Work out the finished part from the listing and answer in its coordinate system (mm). A direction names the side the tool comes from. Round coordinates to 2 decimals unless told otherwise and drop trailing zeros. Loops run counter-clockwise (first coordinate to the right, second up) from the corner with the lowest first, then second, coordinate; pieces in that order, holes last. Notation, with made-up numbers: (-12, 66.5) -> (32, 66.5) arc R24 cw to (32, 89.5) -> close; hole circle Ø1 at (74, -16). An arc over 180 degrees is marked (long way). Write item = value, one per line. Start each with the question number.
```python
from build123d import *

# Parameters (mm, degrees)
BOSS_EXTRU_1_DEPTH      = 7.5
ENL_V_MAT_EXTRU_1_DEPTH = 2
ESQUISSE5_R             = 3.25
ENL_V_MAT_EXTRU_2_DEPTH = 144.052645944
ESQUISSE7_R             = 6.5
ENL_V_MAT_EXTRU_3_DEPTH = 144.143492733


with BuildPart() as part:
    # Esquisse2 → Boss.-Extru.1 (new body)
    with BuildSketch(Plane(origin=(0, 0, 0), x_dir=(1, 0, 0), z_dir=(0, 1, 0))):
        with BuildLine():
            Line((79.497474683, -37.071067812), (42.426406871, 0))
            Line((42.426406871, 0), (79.497474683, 37.071067812))
            ThreePointArc((79.497474683, 37.071067812), (79.497474683, 79.497474683), (37.071067812, 79.497474683))
            Line((37.071067812, 79.497474683), (0, 42.426406871))
            Line((0, 42.426406871), (-37.071067812, 79.497474683))
            ThreePointArc((-37.071067812, 79.497474683), (-79.497474683, 79.497474683), (-79.497474683, 37.071067812))
            Line((-79.497474683, 37.071067812), (-42.426406871, 0))
            Line((-42.426406871, 0), (-79.497474683, -37.071067812))
            ThreePointArc((-79.497474683, -37.071067812), (-79.497474683, -79.497474683), (-37.071067812, -79.497474683))
            Line((-37.071067812, -79.497474683), (-30, -72.426406871))
            Line((-30, -72.426406871), (-30, -82.426406871))
            ThreePointArc((-30, -82.426406871), (0, -112.426406871), (30, -82.426406871))
            Line((30, -82.426406871), (30, -72.426406871))
            Line((30, -72.426406871), (37.071067812, -79.497474683))
            ThreePointArc((37.071067812, -79.497474683), (79.497474683, -79.497474683), (79.497474683, -37.071067812))
        make_face()
    extrude(amount=BOSS_EXTRU_1_DEPTH)

    # Esquisse4 → Enlèv. mat.-Extru.1 (cut)
    with BuildSketch(Plane(origin=(0, 0, 0), x_dir=(-1, 0, 0), z_dir=(0, -1, 0))):
        with BuildLine():
            Line((-33.535533906, -33.535533906), (-18.245921943, -18.245921943))
            Line((-18.245921943, -18.245921943), (-28.852523661, -7.639320225))
            Line((-28.852523661, -7.639320225), (-46.53019319, -25.316989755))
            ThreePointArc((-46.53019319, -25.316989755), (-39.575984314, -28.703872332), (-33.535533906, -33.535533906))
        make_face()
        with BuildLine():
            Line((-7.639320225, -28.852523661), (-18.245921943, -18.245921943))
            Line((-18.245921943, -18.245921943), (-33.535533906, -33.535533906))
            ThreePointArc((-33.535533906, -33.535533906), (-28.703872332, -39.575984314), (-25.316989755, -46.53019319))
            Line((-25.316989755, -46.53019319), (-7.639320225, -28.852523661))
        make_face()
        with BuildLine():
            ThreePointArc((-46.53019319, 25.316989755), (-33.535533906, 33.535533906), (-25.316989755, 46.53019319))
            Line((-25.316989755, 46.53019319), (-7.639320225, 28.852523661))
            Line((-7.639320225, 28.852523661), (-28.852523661, 7.639320225))
            Line((-28.852523661, 7.639320225), (-46.53019319, 25.316989755))
        make_face()
        with BuildLine():
            ThreePointArc((25.316989755, 46.53019319), (33.535533906, 33.535533906), (46.53019319, 25.316989755))
            Line((46.53019319, 25.316989755), (28.852523661, 7.639320225))
            Line((28.852523661, 7.639320225), (7.639320225, 28.852523661))
            Line((7.639320225, 28.852523661), (25.316989755, 46.53019319))
        make_face()
        with BuildLine():
            ThreePointArc((46.53019319, -25.316989755), (33.535533906, -33.535533906), (25.316989755, -46.53019319))
            Line((25.316989755, -46.53019319), (7.639320225, -28.852523661))
            Line((7.639320225, -28.852523661), (28.852523661, -7.639320225))
            Line((28.852523661, -7.639320225), (46.53019319, -25.316989755))
        make_face()
    extrude(amount=-ENL_V_MAT_EXTRU_1_DEPTH, mode=Mode.SUBTRACT)

    # Esquisse5 → Enlèv. mat.-Extru.2 (cut, through all)
    with BuildSketch(Plane(origin=(0, 2, 0), x_dir=(-1, 0, 0), z_dir=(0, -1, 0))):
        with Locations(Location((-25.316989755, -25.316989755, 0), (0, 0, 90))):
            Circle(ESQUISSE5_R)
        with Locations(Location((-25.316989755, 25.316989755, 0), (0, 0, 90))):
            Circle(ESQUISSE5_R)
        with Locations(Location((25.316989755, 25.316989755, 0), (0, 0, 90))):
            Circle(ESQUISSE5_R)
        with Locations(Location((25.316989755, -25.316989755, 0), (0, 0, 90))):
            Circle(ESQUISSE5_R)
    extrude(amount=-ENL_V_MAT_EXTRU_2_DEPTH, mode=Mode.SUBTRACT)

    # Esquisse7 → Enlèv. mat.-Extru.3 (cut, through all)
    with BuildSketch(Plane(origin=(0, 0, 0), x_dir=(-1, 0, 0), z_dir=(0, -1, 0))):
        with Locations(Location((0, -82.426406871, 0), (0, 0, 90))):
            Circle(ESQUISSE7_R)
        with Locations(Location((-58.284271247, -58.284271247, 0), (0, 0, 90))):
            Circle(ESQUISSE7_R)
        with Locations(Location((-58.284271247, 58.284271247, 0), (0, 0, 90))):
            Circle(ESQUISSE7_R)
        with Locations(Location((58.284271247, 58.284271247, 0), (0, 0, 90))):
            Circle(ESQUISSE7_R)
        with Locations(Location((58.284271247, -58.284271247, 0), (0, 0, 90))):
            Circle(ESQUISSE7_R)
    extrude(amount=-ENL_V_MAT_EXTRU_3_DEPTH, mode=Mode.SUBTRACT)


solid = part.part
```
Item 1: Section D-D (x = 68.5) is taken. Determine the outline of the cut face in (y, z), then the cut area to 3 significant figures.
Item 2: A tool of negligible diameter and unlimited length cuts with its end or side. For faces 1 (the flat face through (-60.702, 3.698, 18.276)), 2 (the flat face through (18.1, 0.99, -18.39)), 3 (the flat face through (-18.276, 3.698, -60.702)), from which of +Z, -Z, +X, -X, +Y, -Y can it reach the whole face along a straight path? Write none if from no direction.
Item 3: Section C-C (x = 15.5) is taken. Determine the outline of the cut face in (y, z).
Item 4: Section B-B (y = 6) is taken. Count the separate pieces of the cut face and the enclosed holes in it, then the cut area to 3 significant figures.
Item 5: The mould has two halves that part along X. Classify faces 4 (the flat face through (-61.221, 3.698, -18.795)), 5 (the cylindrical face through (-33.38, 0.99, -33.69)): pulls with the +X half, pulls with the -X half, needs draft (parallel to the pull), parting line crosses it, or undercut.
Item 6: Flat-ended cylindrical pins translate along their axes: pin 1 (2 mm diameter, centred on x = -0.5, y = 4.5, fed in from -Z); pin 2 (4 mm diameter, centred on x = 25.32, z = 25.32, fed in from -Y); pin 3 (4 mm diameter, centred on y = 2.5, z = 75, fed in from +X); pin 4 (19.5 mm diameter, centred on x = -25.5, z = 27.5, fed in from -Y). Find the tip coordinate at first contact, or state that the pin passes through.
Item 7: Find the intervals of material crossed by line 1 along Z through (x, y) = (-54, 5); line 2 along Z through (x, y) = (-27.5, 3.5); line 3 along X through (y, z) = (6.75, 75), in increasing order. Write a range as [from, to].
Item 8: Section A-A (x = -74) is taken. Determine the outline of the cut face in (y, z).
Worked answers:
q1.outline = (0, -86.49) -> (7.5, -86.49) -> (7.5, -26.07) -> (0, -26.07) -> close; (0, 26.07) -> (7.5, 26.07) -> (7.5, 86.49) -> (0, 86.49) -> close
q1.area = 906 mm2
q2.face_1 = -X, +Y, -Y
q2.face_2 = -Y
q2.face_3 = -Z, +Y, -Y
q3.outline = (0, -57.93) -> (7.5, -57.93) -> (7.5, 108.11) -> (0, 108.11) -> (0, 36.71) -> (2, 36.71) -> (2, 20.99) -> (0, 20.99) -> (0, -20.99) -> (2, -20.99) -> (2, -36.71) -> (0, -36.71) -> close
q4.separate_pieces = 1
q4.enclosed_holes = 9
q4.area = 24,000 mm2
q5.face_4 = pulls with the -X half
q5.face_5 = undercut
q6.pin_1 = -43.93
q6.pin_2 = through
q6.pin_3 = 84.43
q6.pin_4 = 2
q7.line_1 = [-87.98, -63.17], [-53.4, -11.57], [11.57, 53.4], [63.17, 87.98]
q7.line_2 = [-69.93, -27.72], [-22.91, 22.91], [27.72, 94.42]
q7.line_3 = [-83.2, -32.57], [-30, 30], [32.57, 83.2]
q8.outline = (0, -83.84) -> (7.5, -83.84) -> (7.5, -31.57) -> (0, -31.57) -> close; (0, 31.57) -> (7.5, 31.57) -> (7.5, 83.84) -> (0, 83.84) -> close
